Check sheet for the modelled part. Datum: model origin and axes. Units: mm. A direction names the side the tool comes from. Give positions to 0.01 mm unless a question says otherwise; leave off trailing zeros. Order: outer loops, then holes, each group sorted by start corner. A loop starts at its lowest first (then second) coordinate and runs counter-clockwise, first axis right, second up.
Item 1: Sectioned sample at D-D on x = -22.5. Record the boundary of the cut face in (y, z), and give its area (3 significant figures).
Item 2: Release check for a two-part mould opening along Z. For faces 1 (the cylindrical face through (-0.168, 19.544, 40.853)), 2 (the cylindrical face through (-14.14, -19.1, 51.59)), 3 (the flat face through (0, 6, 13)) record: released by +Z, released by -Z, zero draft, split by the parting line, or undercut.
Item 3: Sectioned sample at B-B on x = 0. Count the separate pieces of the cut face and the enclosed holes in it, and give its area (3 significant figures).
Item 4: Material ranges on line 1 along X through (y, z) = (11.75, 60); line 2 along Z through (x, y) = (0.5, -10.5); line 3 along Z through (x, y) = (0, -11), recorded low to high.
Item 5: Sectioned sample at C-C on z = 49.5. Record the boundary of the cut face in (x, y).
Item 6: Sectioned sample at A-A on y = 0. Record the boundary of the cut face in (x, z).
Item 7: Gauge pin test, flat ends, axial feed: P1, Ø7.5, axis at x = 23.88, y = 0, coming from the +Z side; P2, Ø1.8, axis at x = 4.5, z = -4.5, coming from the -Y side; P3, Ø3, axis at x = -6, z = -2.5, coming from the +Y side; P4, Ø19, axis at x = -4.5, z = 13, coming from the -Y side. Record the tip position at first contact, or that the pin passes through.
Item 8: Access from +Z, -Z, +X, -X, +Y, -Y to the whole of each face (thin tool, end or side, straight path). Record for faces 4 (the flat face through (-15, 2, 39)), 5 (the cylindrical face through (14.14, -5.1, 13.08)), 6 (the flat face through (0, 12.5, -3)), 7 (the flat face through (0, 8, 68)).
Autodesk Inventor part; units mm, degrees
ref_plane "YZ Plane" through (0, 0, 0) normal (1, 0, 0) x (0, 1, 0)
ref_plane "XZ Plane" through (0, 0, 0) normal (0, 1, 0) x (-1, 0, 0)
ref_plane "XY Plane" through (0, 0, 0) normal (0, 0, 1) x (1, 0, 0)
sketch "Sketch1" plane through (0, 0, 0) normal (0, 1, 0) x (-1, 0, 0)
  arc A0 (15, 60) -> (-15, 60) centre (0, 60) ccw
  line L0 (-15, 60) -> (-15, 0)
  line L1 (-15, 0) -> (15, 0)
  line L2 (15, 0) -> (15, 60)
  line L3 (21, 0) -> (-21, 0)
  line L4 (0, -15) -> (0, 90)
  circle A1 centre (0, 60) radius 6.7766
  point P0 (0, 0)
  dimension "d0" = 30
  dimension "d1" = 60
  dimension "d2" = 15
extrude "Extrusion1" add sketch "Sketch1" along normal mid plane 40 contours L2 L1 L4 A1 A0 | L4 A1 L1 L0 A0
sketch "Sketch2" plane through (15, -20, 0) normal (1, 0, 0) x (0, 0, -1)
  line L0 (0, 0) -> (0, 40)
  line L1 (-60, 40) -> (0, 40)
  line L2 (0, 0) -> (-60, 0)
  line L3 (-60, 40) -> (-60, 40)
  line L4 (-60, 0) -> (-60, 0)
  line L5 (-75, 0) -> (-75, 40)
  line L6 (-75, 12) -> (-51.3579, 12)
  line L7 (-51.3579, 28) -> (-75, 28)
  line L8 (-75, 28) -> (-75, 12)
  line L9 (-53.2234, 0) -> (-66.7766, 0)
  line L10 (-93.6547, 20) -> (5.2074, 20) construction
  line L11 (-40.607, 0) -> (-28.8596, 14)
  line L12 (-28.8596, 14) -> (0, 14)
  line L13 (0, 0) -> (0, 40) construction
  line L14 (-40.607, 40) -> (-28.8596, 26)
  line L15 (-28.8596, 26) -> (0, 26)
  line L16 (0, 0) -> (-60, 0) construction
  line L17 (-60, 40) -> (0, 40) construction
  arc A0 (-51.3579, 12) -> (-51.3579, 28) centre (-51.3579, 20) ccw
  line L18 (-53.2234, 0) -> (-66.7766, 0)
  line L19 (-66.7766, 40) -> (-53.2234, 40)
  line L20 (-53.2234, 40) -> (-53.2234, 0)
  point P0 (0, 20)
  point P1 (-75, 20)
  point P2 (0, 20)
  point P3 (-40.607, 0)
  dimension "d5" = 130
  dimension "d6" = 12
  dimension "d7" = 16
  dimension "d8" = 8
extrude "Extrusion2" cut sketch "Sketch2" against normal blind 40 contours L2 L11 L12 L0 | L15 L14 L1 L0 | L20 L7 A0 L6 | L6 L5 L7 L20
fillet "Fillet1" radius 5 4 edges at (0, -20, 40.607) (0, -6, 28.8596) (0, 6, 28.8596) (0, 20, 40.607)
fillet "Fillet2" radius 3 22 edges at (-15, -20, 51.4693) (-15, -19.5315, 40.8254) (-15, -13, 34.7333) (-15, -6.4685, 28.6411) (-15, -6, 13.264) (15, -20, 51.4693) (15, -19.5315, 40.8254) (15, -13, 34.7333) (15, -6.4685, 28.6411) (15, -6, 13.264) (0, -20, 75) (15, 20, 51.4693) (15, 19.5315, 40.8254) (15, 13, 34.7333) (15, 6.4685, 28.6411) (15, 6, 13.264) (-15, 20, 51.4693) (-15, 19.5315, 40.8254) (-15, 13, 34.7333) (-15, 6.4685, 28.6411) (-15, 6, 13.264) (0, 20, 75)
sketch "Sketch3" plane through (12, -6, 0) normal (0, 0, -1) x (-1, 0, 0)
  arc A0 (0, 12) -> (-3, 9) centre (0, 9) ccw
  line L0 (-3, 3) -> (-3, 9)
  arc A1 (-3, 3) -> (0, 0) centre (0, 3) ccw
  line L1 (0, 0) -> (24, 0)
  arc A2 (24, 0) -> (27, 3) centre (24, 3) ccw
  line L2 (27, 9) -> (27, 3)
  arc A3 (27, 9) -> (24, 12) centre (24, 9) ccw
  line L3 (24, 12) -> (0, 12)
  line L4 (-11.8816, 6) -> (35.8816, 6) construction
  line L5 (-11.8816, -6.5) -> (35.8816, -6.5)
  line L6 (35.8816, 18.5) -> (-11.8816, 18.5)
  arc A4 (-11.8816, 18.5) -> (-11.8816, -6.5) centre (-11.8816, 6) ccw
  arc A5 (35.8816, -6.5) -> (35.8816, 18.5) centre (35.8816, 6) ccw
  circle A6 centre (35.8816, 6) radius 4.0304
  circle A7 centre (-11.8816, 6) radius 4.0304
  point P0 (12, 6)
  point P1 (12, 6)
  dimension "d13" = 25
extrude "Extrusion3" add sketch "Sketch3" along normal blind 6 contours L3 A3 L2 A2 L1 A1 L0 A0 | A4 L6 A5 L5
properties part number "Fitting"
Report:
1. outline: (-12.5, -6) - (-3.79, -6) - (-3.79, 0) - (-12.5, 0) - close; (3.79, -6) - (12.5, -6) - (12.5, 0) - (3.79, 0) - close
1. area: 105 mm2
2. face 1: released by -Z
2. face 2: zero draft
2. face 3: undercut
3. separate pieces: 3
3. enclosed holes: 0
3. area: 1,370 mm2
4. line 1: x = -15 to -6.78, 6.78 to 15
4. line 2: z = -6 to 0, 32.64 to 53.24, 66.76 to 74.99
4. line 3: z = -6 to 0, 33.06 to 53.22, 66.78 to 75
5. outline: (-15, -17) arc R3 ccw to (-12, -20) - (12, -20) arc R3 ccw to (15, -17) - (15, -7.78) - (-15, -7.78) - close; (-15, 7.78) - (15, 7.78) - (15, 17) arc R3 ccw to (12, 20) - (-12, 20) arc R3 ccw to (-15, 17) - close
6. outline: (-36.38, -6) - (-27.91, -6) - (-27.91, 0) - (-36.38, 0) - close; (-19.85, -6) - (19.85, -6) - (19.85, 0) - (15, 0) - (15, 43.36) - (-15, 43.36) - (-15, 0) - (-19.85, 0) - close; (27.91, -6) - (36.38, -6) - (36.38, 0) - (27.91, 0) - close
7. P1: passes through
7. P2: stops at y = -12.5
7. P3: stops at y = 12.5
7. P4: stops at y = -6
8. face 4: +Z, -X, +Y, -Y
8. face 5: +X, -Y
8. face 6: -Z, +X, -X, +Y
8. face 7: +Z, +X, -X
